```python
from build123d import *

# Parameters (mm, degrees)
CROQUIS1_W              = 35
CROQUIS1_H              = 25.2
SALIENTE_EXTRUIR1_DEPTH = 9
CORTAR_EXTRUIR1_DEPTH   = 10
CROQUIS3_W              = 17.198072292
CROQUIS3_H              = 25.2
CORTAR_EXTRUIR2_DEPTH   = 10


with BuildPart() as part:
    # Croquis1 → Saliente-Extruir1 (new body)
    with BuildSketch(Plane(origin=(0, 0, 0), x_dir=(1, 0, 0), z_dir=(0, 1, 0))):
        Rectangle(CROQUIS1_W, CROQUIS1_H)
    extrude(amount=SALIENTE_EXTRUIR1_DEPTH)

    # Croquis2 → Cortar-Extruir1 (cut, through all)
    with BuildSketch(Plane.XZ):
        with BuildLine():
            Line((-4.457181896, 2.743708499), (-4.457181896, 8.743708499))
            ThreePointArc((-4.457181896, 8.743708499), (-2.907181896, 10.293708499), (-1.357181896, 8.743708499))
            Line((-1.357181896, 8.743708499), (-1.357181896, 2.743708499))
            ThreePointArc((-1.357181896, 2.743708499), (-2.907181896, 1.193708499), (-4.457181896, 2.743708499))
        make_face()
        with BuildLine():
            Line((-12.740890395, -8.64), (-12.740890395, -2.64))
            ThreePointArc((-12.740890395, -2.64), (-14.290890395, -1.09), (-15.840890395, -2.64))
            Line((-15.840890395, -2.64), (-15.840890395, -8.64))
            ThreePointArc((-15.840890395, -8.64), (-14.290890395, -10.19), (-12.740890395, -8.64))
        make_face()
    extrude(amount=-CORTAR_EXTRUIR1_DEPTH, mode=Mode.SUBTRACT)

    # Croquis3 → Cortar-Extruir2 (cut, through all)
    with BuildSketch(Plane.XZ):
        with Locations((8.900963854, 0)):
            Rectangle(CROQUIS3_W, CROQUIS3_H)
    extrude(amount=-CORTAR_EXTRUIR2_DEPTH, mode=Mode.SUBTRACT)


solid = part.part
```
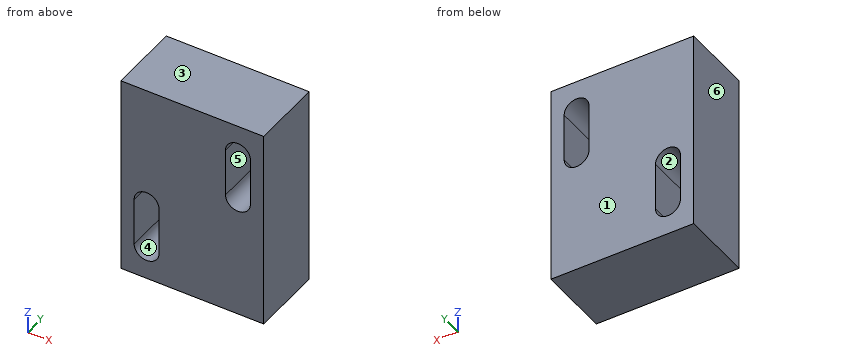
Work out the finished part from the listing and answer in its coordinate system (mm). Face numbers are marked on the shaded views. A direction names the side the tool comes from. Give positions to 0.01 mm unless a question says otherwise; leave off trailing zeros. Order: outer loops, then holes, each group sorted by start corner. A loop starts at its lowest first (then second) coordinate and runs counter-clockwise, first axis right, second up. Notation, with made-up numbers: M 68.25,46 L 100.25,46 A16 cw 100.25,51 Z; hole C 28.25,-1 d7. An arc over 180 degrees is marked long. Return JSON: item names as keys, results as strings.
1) Straight lines are drawn through the part: line 1 along Z through (x, y) = (-3, 7); line 2 along X through (y, z) = (3.5, 8); line 3 along X through (y, z) = (5.25, -6.75). For each, find the intervals that lie inside material, in ascending order. Write a range as [from, to].
Resolved:
{"line 1": "[-12.6, 1.2], [10.29, 12.6]", "line 2": "[-17.5, -4.46], [-1.36, 0.3]", "line 3": "[-17.5, -15.84], [-12.74, 0.3]"}
2) A tool of negligible diameter and unlimited length cuts with its end or side. For the marked faces 1 and 2, from which of +Z, -Z, +X, -X, +Y, -Y can it reach the whole face along a straight path? Write none if from no direction.
Resolved:
{"face 1": "+Z, -Z, +X, -X, +Y", "face 2": "+Y, -Y"}
3) Section B-B, the plane y = 7.75 is taken. Write down the section's boundary in (x, z), plus the area to 3 significant figures.
Resolved:
{"outline": "M -17.5,-12.6 L 0.3,-12.6 L 0.3,12.6 L -17.5,12.6 Z; hole M -15.84,-8.64 A1.55 ccw -12.74,-8.64 L -12.74,-2.64 A1.55 ccw -15.84,-2.64 Z; hole M -4.46,2.74 A1.55 ccw -1.36,2.74 L -1.36,8.74 A1.55 ccw -4.46,8.74 Z", "area": "396 mm^2"}
4) Section C-C, the plane z = 10 is taken. Write down the section's boundary in (x, y).
Resolved:
{"outline": "M -17.5,0 L -3.82,0 L -3.82,9 L -17.5,9 Z; M -2,0 L 0.3,0 L 0.3,9 L -2,9 Z"}
5) For a pull along Z with two mould halves and no side action, classify the marked faces 3, 4, 5 and 6 as +Z half, -Z half, draft (parallel to the pull), parting line (faces both ways), or undercut.
Resolved:
{"face 3": "+Z half", "face 4": "undercut", "face 5": "undercut", "face 6": "draft"}
6) Section A-A, the plane x = -3.75 is taken. Write down the section's boundary in (y, z).
Resolved:
{"outline": "M 0,-12.6 L 9,-12.6 L 9,1.44 L 0,1.44 Z; M 0,10.04 L 9,10.04 L 9,12.6 L 0,12.6 Z"}
7) This flat-tipped pin is pushed along its axis until it touches: pin 1 (4 mm diameter, centred on x = -7, z = 10, fed in from -Y). Where does it stop, or does it pass through?
Resolved:
{"pin 1": "y = 0"}
